```python
from build123d import *

# Parameters (mm, degrees)
F0_R     = 12
F1_DEPTH = 25
F4_R     = 17.5
F4_R_2   = 12
F5_DEPTH = 0.8
F6_SIZE  = 2.5


with BuildPart() as f1:
    # F0 (on Front) → F1 (new body)
    with BuildSketch(Plane.XZ):
        Polygon((11.547005, -20), (23.094011, 0), (11.547005, 20), (-11.547005, 20), (-23.094011, 0), (-11.547005, -20), align=None)
        Circle(F0_R, mode=Mode.SUBTRACT)
    extrude(amount=F1_DEPTH)

    # F2 (on Top) → F3 (revolve, cut)
    with BuildSketch(Plane.XY):
        Polygon((31.622065, 2.590499), (18, 0), (34.060234, -9.272381), align=None)
    revolve(axis=Axis((0, -9.323449, 0), (0, 1, 0)), mode=Mode.SUBTRACT)

    # F4 (on face) → F5 (join)
    with BuildSketch(Plane.XZ.offset(25)):
        Circle(F4_R)
        Circle(F4_R_2, mode=Mode.SUBTRACT)
    extrude(amount=F5_DEPTH)

    # F6
    f6_edges = [f1.edges().sort_by_distance(p)[0] for p in [
        (-12, -25.8, 0),
        (-12, 0, 0),
    ]]
    chamfer(f6_edges, length=F6_SIZE)


solid = f1.part
```
Input: part model. Units: mm. Frame: model coordinates. A direction names the side the tool comes from. Give positions to 0.01 mm unless a question says otherwise; leave off trailing zeros. Loops run counter-clockwise (first coordinate to the right, second up) from the corner with the lowest first, then second, coordinate; pieces in that order, holes last. Notation, with made-up numbers: M 36,3 L 40,3 A15 ccw 40,21 Z; hole C 68.5,78 d2. An arc over 180 degrees is marked long. Answer as CSV lines item,"result". Start each with the question number.
1. Line query: L1, parallel to Z at x = 0, y = -14.75; L2, parallel to Z at x = 8, y = -6; L3, parallel to X at y = -18, z = 4. Output: solid intervals per line, ascending.
2. Section A-A on y = -19. Return loops of the section in (x, z), plus the area to 3 significant figures.
3. Pin query (flat end, axial travel): P1, Ø19, axis at x = 0, z = 0, coming from the -Y side; P2, Ø4, axis at x = -8.5, z = 7, coming from the -Y side; P3, Ø5, axis at y = -12, z = -6.5, coming from the -X side; P4, Ø3, axis at y = -20, z = -7, coming from the -X side. Return the tip coordinate at first contact, or that it passes through.
4. Section B-B on x = 0. Return loops of the section in (y, z).
5. Reachability of faces 4 (the face through (17, -25, 5)), 5 (the face through (17.4, -12.91, 9.86)) from +Z, -Z, +X, -X, +Y, -Y: full face, straight path, thin tool, end or side. Return the list, or none.
6. Pull-direction query (Z, two-part tool) for faces 1 (the face through (16.922, -0.184, 7.016)), 2 (the face through (-7, -25.8, 13)), 3 (the face through (-11.99, -12.75, 0.53)); classes: released by +Z, released by -Z, zero draft, split by the parting line, or undercut.
Computed values:
1,L1,"z = -20 to -12, 12 to 20"
1,L2,"z = -20 to -8.94, 8.94 to 20"
1,L3,"x = -20.78 to -11.31, 11.31 to 20.78"
2,outline,"M -23.09,0 L -11.55,-20 L 11.55,-20 L 23.09,0 L 11.55,20 L -11.55,20 Z; hole C 0,0 d24"
2,area,"933 mm²"
3,P1,"passes through"
3,P2,"stops at y = -24.31"
3,P3,"stops at x = -20.78"
3,P4,"stops at x = -19.92"
4,outline,"M -25.8,-17.5 L -25,-17.5 L -25,-20 L -1.15,-20 L 0,-18 L 0,-14.5 L -2.5,-12 L -23.3,-12 L -25.8,-14.5 Z; M -25.8,14.5 L -23.3,12 L -2.5,12 L 0,14.5 L 0,18 L -1.15,20 L -25,20 L -25,17.5 L -25.8,17.5 Z"
5,face 4,"-Y"
5,face 5,"+Z, +X, +Y, -Y"
6,face 1,"split by the parting line"
6,face 2,"zero draft"
6,face 3,"undercut"
